from build123d import *

# Parameters (mm, degrees)
F0_R     = 6.75
F1_DEPTH = 3.175
F2_R     = 9.75
F3_DEPTH = 2.1
F4_SIZE  = 1
F5_T     = -2


with BuildPart() as f1:
    # F0 (on Top) → F1 (new body)
    with BuildSketch(Plane.XY):
        Circle(F0_R)
    extrude(amount=F1_DEPTH)

    # F2 (on face) → F3 (join)
    with BuildSketch(Plane.XY.offset(3.175)):
        Circle(F2_R)
    extrude(amount=F3_DEPTH)

    # F4
    f4_edges = [f1.edges().sort_by_distance(p)[0] for p in [
        (-9.75, 0, 5.275),
    ]]
    chamfer(f4_edges, length=F4_SIZE)

    # F5
    f5_openings = [f1.faces().sort_by_distance(p)[0] for p in [
        (0, 0, 0),
    ]]
    offset(amount=F5_T, openings=f5_openings, kind=Kind.INTERSECTION)


solid = f1.part
Check sheet for the modelled part. Datum: model origin and axes. Units: mm. A direction names the side the tool comes from. Round coordinates to 2 decimals unless told otherwise and drop trailing zeros. Write each loop counter-clockwise with the first axis right and the second up, starting at its lowest first coordinate (ties: lowest second). Pieces come first, ordered by that corner, then holes. Notation, with made-up numbers: (28, 25) - (49, 25) arc R21 ccw to (49, 45) - close; hole circle Ø4 at (49, 6). An arc over 180 degrees is marked (long way). Return JSON: item names as keys, results as strings.
Q1. Cross-section at A-A (x = 0). Record the boundary of the cut face in (y, z) (3 decimals), then the cut area to 3 significant figures.
Returned:
{"outline": "(-9.75, 3.175) - (-6.75, 3.175) - (-6.75, 0) - (-4.75, 0) - (-4.75, 3.275) - (4.75, 3.275) - (4.75, 0) - (6.75, 0) - (6.75, 3.175) - (9.75, 3.175) - (9.75, 4.275) - (8.75, 5.275) - (-8.75, 5.275) - (-9.75, 4.275) - close", "area": "51.7 mm²"}
Q2. Depth check by flat-ended pin: P1, Ø1.5, axis at x = 4, z = 3, coming from the +Y side. Enter the tip coordinate at first touch or a pass-through.
Returned:
{"P1": "stops at y = 9.19"}
Q3. Scan lines: L1, parallel to Y at x = 0, z = 2.5; L2, parallel to Z at x = 1.5, y = -7.5 (3 decimals); L3, parallel to X at y = 4.25, z = 2.9. Record each from-to range of solid material in increasing order. Write a range as from..to.
Returned:
{"L1": "y = -6.75..-4.75, 4.75..6.75", "L2": "z = 3.175..5.275", "L3": "x = -5.24..-2.12, 2.12..5.24"}
Q4. Draft check along Y on faces 1 (the flat face through (0, 0, 5.275)), 2 (the cylindrical face through (2.192, -4.214, 1.615)), 3 (the cylindrical face through (-1.269, 9.667, 3.717)). Enter one of: released by +Y, released by -Y, zero draft, split by the parting line, or undercut.
Returned:
{"face 1": "zero draft", "face 2": "undercut", "face 3": "split by the parting line"}
Q5. Cross-section at C-C (z = 1.15). Record the boundary of the cut face in (x, y), then the cut area to 3 significant figures.
Returned:
{"outline": "circle Ø13.5 at (0, 0); hole circle Ø9.5 at (0, 0)", "area": "72.3 mm²"}
Q6. Cross-section at D-D (z = 4.55). Record the boundary of the cut face in (x, y) (3 decimals).
Returned:
{"outline": "circle Ø18.95 at (0, 0)"}
Q7. Access from +Z, -Z, +X, -X, +Y, -Y to the whole of each face (thin tool, end or side, straight path). Record for faces 4 (the flat face through (0, 0, 3.275)), 5 (the flat face through (1, 5, 0)).
Returned:
{"face 4": "-Z", "face 5": "-Z, +X, -X, +Y, -Y"}
